from build123d import *
from OCP.BRepFilletAPI import BRepFilletAPI_MakeChamfer

# Parameters (mm, degrees)
BOSS_EXTRUDE1_DEPTH         = 2.29
SKETCH3_W                   = 0.64
SKETCH3_H                   = 0.64
CHAMFER3_SIZE               = 0.5
CHAMFER3_SIZE2              = 0.133974596
LPATTERN1_COUNT             = 6
LPATTERN1_PITCH             = 2.54
CHAMFER3_OF_LPATTERN1_SIZE  = 0.5
CHAMFER3_OF_LPATTERN1_SIZE2 = 0.133974596


with BuildPart() as part:
    # Sketch1 → Boss-Extrude1 (new body)
    with BuildSketch(Plane(origin=(0, 0, 0), x_dir=(1, 0, 0), z_dir=(0, 1, 0))):
        Polygon((-0.77, 1.25), (0.77, 1.25), (1.25, 0.75), (1.27, 0.75), (1.27, -0.75), (1.25, -0.75), (0.77, -1.25), (-0.77, -1.25), (-1.25, -0.75), (-1.27, -0.75), (-1.27, 0.75), (-1.25, 0.75), align=None)
    boss_extrude1 = extrude(amount=BOSS_EXTRUDE1_DEPTH)

    # Sweep1: sweep along a path in Sketch2
    with BuildLine(Plane(origin=(0, 0, 0), x_dir=(0, 0, -1), z_dir=(1, 0, 0))) as sweep1_path:
        Line((0, 17.12), (0, -0.408142235))
        ThreePointArc((0, -0.408142235), (-0.152240935, -1.1735091), (-0.585786438, -1.822355798))
        Line((-0.585786438, -1.822355798), (-5.26343064, -6.5))
    # Sketch3 → Sweep1 (sweep)
    with BuildSketch(Plane(origin=(0, 17.12, 0), x_dir=(1, 0, 0), z_dir=(0, 1, 0))):
        Rectangle(SKETCH3_W, SKETCH3_H)
    sweep1 = sweep(path=sweep1_path.line)

    # Chamfer3: one chamfer whose edges measure the first distance from different faces: ONE call of the kernel's chamfer builder (chamfer() names one face for all edges)
    chamfer3_edges_1 = [part.edges().sort_by_distance(p)[0] for p in [
        (0.32, 17.12, 0),
    ]]
    chamfer3_side_1 = [part.faces().sort_by_distance(p)[0] for p in [
        (0.32, 9.705, 0),
    ]]
    chamfer3_edges_2 = [part.edges().sort_by_distance(p)[0] for p in [
        (0, 17.12, -0.32),
    ]]
    chamfer3_side_2 = [part.faces().sort_by_distance(p)[0] for p in [
        (0, 9.705, -0.32),
    ]]
    chamfer3_edges_3 = [part.edges().sort_by_distance(p)[0] for p in [
        (-0.32, 17.12, 0),
    ]]
    chamfer3_side_3 = [part.faces().sort_by_distance(p)[0] for p in [
        (-0.32, 9.705, 0),
    ]]
    chamfer3_edges_4 = [part.edges().sort_by_distance(p)[0] for p in [
        (0, 17.12, 0.32),
    ]]
    chamfer3_side_4 = [part.faces().sort_by_distance(p)[0] for p in [
        (0, 9.705, 0.32),
    ]]
    chamfer3 = BRepFilletAPI_MakeChamfer(part.part.solid().wrapped)
    for e in chamfer3_edges_1:
        chamfer3.Add(CHAMFER3_SIZE, CHAMFER3_SIZE2, e.wrapped, chamfer3_side_1[0].wrapped)  # the first distance lies on this face
    for e in chamfer3_edges_2:
        chamfer3.Add(CHAMFER3_SIZE, CHAMFER3_SIZE2, e.wrapped, chamfer3_side_2[0].wrapped)  # the first distance lies on this face
    for e in chamfer3_edges_3:
        chamfer3.Add(CHAMFER3_SIZE, CHAMFER3_SIZE2, e.wrapped, chamfer3_side_3[0].wrapped)  # the first distance lies on this face
    for e in chamfer3_edges_4:
        chamfer3.Add(CHAMFER3_SIZE, CHAMFER3_SIZE2, e.wrapped, chamfer3_side_4[0].wrapped)  # the first distance lies on this face
    add(Compound.cast(chamfer3.Shape()), mode=Mode.REPLACE)

    # LPattern1: Boss-Extrude1, Sweep1 ×6
    with Locations(*[(i * LPATTERN1_PITCH, 0, 0) for i in range(1, LPATTERN1_COUNT)]):
        add(boss_extrude1)
        add(sweep1)

    # Chamfer3 of LPattern1: one chamfer whose edges measure the first distance from different faces: ONE call of the kernel's chamfer builder (chamfer() names one face for all edges)
    chamfer3_of_lpattern1_edges_1 = [part.edges().sort_by_distance(p)[0] for p in [
        (2.86, 17.12, 0),
    ]]
    chamfer3_of_lpattern1_side_1 = [part.faces().sort_by_distance(p)[0] for p in [
        (2.86, 9.705, 0),
    ]]
    chamfer3_of_lpattern1_edges_2 = [part.edges().sort_by_distance(p)[0] for p in [
        (2.54, 17.12, -0.32),
    ]]
    chamfer3_of_lpattern1_side_2 = [part.faces().sort_by_distance(p)[0] for p in [
        (2.54, 9.705, -0.32),
    ]]
    chamfer3_of_lpattern1_edges_3 = [part.edges().sort_by_distance(p)[0] for p in [
        (2.22, 17.12, 0),
    ]]
    chamfer3_of_lpattern1_side_3 = [part.faces().sort_by_distance(p)[0] for p in [
        (2.22, 9.705, 0),
    ]]
    chamfer3_of_lpattern1_edges_4 = [part.edges().sort_by_distance(p)[0] for p in [
        (2.54, 17.12, 0.32),
    ]]
    chamfer3_of_lpattern1_side_4 = [part.faces().sort_by_distance(p)[0] for p in [
        (2.54, 9.705, 0.32),
    ]]
    chamfer3_of_lpattern1_edges_5 = [part.edges().sort_by_distance(p)[0] for p in [
        (5.4, 17.12, 0),
    ]]
    chamfer3_of_lpattern1_side_5 = [part.faces().sort_by_distance(p)[0] for p in [
        (5.4, 9.705, 0),
    ]]
    chamfer3_of_lpattern1_edges_6 = [part.edges().sort_by_distance(p)[0] for p in [
        (5.08, 17.12, -0.32),
    ]]
    chamfer3_of_lpattern1_side_6 = [part.faces().sort_by_distance(p)[0] for p in [
        (5.08, 9.705, -0.32),
    ]]
    chamfer3_of_lpattern1_edges_7 = [part.edges().sort_by_distance(p)[0] for p in [
        (4.76, 17.12, 0),
    ]]
    chamfer3_of_lpattern1_side_7 = [part.faces().sort_by_distance(p)[0] for p in [
        (4.76, 9.705, 0),
    ]]
    chamfer3_of_lpattern1_edges_8 = [part.edges().sort_by_distance(p)[0] for p in [
        (5.08, 17.12, 0.32),
    ]]
    chamfer3_of_lpattern1_side_8 = [part.faces().sort_by_distance(p)[0] for p in [
        (5.08, 9.705, 0.32),
    ]]
    chamfer3_of_lpattern1_edges_9 = [part.edges().sort_by_distance(p)[0] for p in [
        (7.94, 17.12, 0),
    ]]
    chamfer3_of_lpattern1_side_9 = [part.faces().sort_by_distance(p)[0] for p in [
        (7.94, 9.705, 0),
    ]]
    chamfer3_of_lpattern1_edges_10 = [part.edges().sort_by_distance(p)[0] for p in [
        (7.62, 17.12, -0.32),
    ]]
    chamfer3_of_lpattern1_side_10 = [part.faces().sort_by_distance(p)[0] for p in [
        (7.62, 9.705, -0.32),
    ]]
    chamfer3_of_lpattern1_edges_11 = [part.edges().sort_by_distance(p)[0] for p in [
        (7.3, 17.12, 0),
    ]]
    chamfer3_of_lpattern1_side_11 = [part.faces().sort_by_distance(p)[0] for p in [
        (7.3, 9.705, 0),
    ]]
    chamfer3_of_lpattern1_edges_12 = [part.edges().sort_by_distance(p)[0] for p in [
        (7.62, 17.12, 0.32),
    ]]
    chamfer3_of_lpattern1_side_12 = [part.faces().sort_by_distance(p)[0] for p in [
        (7.62, 9.705, 0.32),
    ]]
    chamfer3_of_lpattern1_edges_13 = [part.edges().sort_by_distance(p)[0] for p in [
        (10.48, 17.12, 0),
    ]]
    chamfer3_of_lpattern1_side_13 = [part.faces().sort_by_distance(p)[0] for p in [
        (10.48, 9.705, 0),
    ]]
    chamfer3_of_lpattern1_edges_14 = [part.edges().sort_by_distance(p)[0] for p in [
        (10.16, 17.12, -0.32),
    ]]
    chamfer3_of_lpattern1_side_14 = [part.faces().sort_by_distance(p)[0] for p in [
        (10.16, 9.705, -0.32),
    ]]
    chamfer3_of_lpattern1_edges_15 = [part.edges().sort_by_distance(p)[0] for p in [
        (9.84, 17.12, 0),
    ]]
    chamfer3_of_lpattern1_side_15 = [part.faces().sort_by_distance(p)[0] for p in [
        (9.84, 9.705, 0),
    ]]
    chamfer3_of_lpattern1_edges_16 = [part.edges().sort_by_distance(p)[0] for p in [
        (10.16, 17.12, 0.32),
    ]]
    chamfer3_of_lpattern1_side_16 = [part.faces().sort_by_distance(p)[0] for p in [
        (10.16, 9.705, 0.32),
    ]]
    chamfer3_of_lpattern1_edges_17 = [part.edges().sort_by_distance(p)[0] for p in [
        (13.02, 17.12, 0),
    ]]
    chamfer3_of_lpattern1_side_17 = [part.faces().sort_by_distance(p)[0] for p in [
        (13.02, 9.705, 0),
    ]]
    chamfer3_of_lpattern1_edges_18 = [part.edges().sort_by_distance(p)[0] for p in [
        (12.7, 17.12, -0.32),
    ]]
    chamfer3_of_lpattern1_side_18 = [part.faces().sort_by_distance(p)[0] for p in [
        (12.7, 9.705, -0.32),
    ]]
    chamfer3_of_lpattern1_edges_19 = [part.edges().sort_by_distance(p)[0] for p in [
        (12.38, 17.12, 0),
    ]]
    chamfer3_of_lpattern1_side_19 = [part.faces().sort_by_distance(p)[0] for p in [
        (12.38, 9.705, 0),
    ]]
    chamfer3_of_lpattern1_edges_20 = [part.edges().sort_by_distance(p)[0] for p in [
        (12.7, 17.12, 0.32),
    ]]
    chamfer3_of_lpattern1_side_20 = [part.faces().sort_by_distance(p)[0] for p in [
        (12.7, 9.705, 0.32),
    ]]
    chamfer3_of_lpattern1 = BRepFilletAPI_MakeChamfer(part.part.solid().wrapped)
    for e in chamfer3_of_lpattern1_edges_1:
        chamfer3_of_lpattern1.Add(CHAMFER3_OF_LPATTERN1_SIZE, CHAMFER3_OF_LPATTERN1_SIZE2, e.wrapped, chamfer3_of_lpattern1_side_1[0].wrapped)  # the first distance lies on this face
    for e in chamfer3_of_lpattern1_edges_2:
        chamfer3_of_lpattern1.Add(CHAMFER3_OF_LPATTERN1_SIZE, CHAMFER3_OF_LPATTERN1_SIZE2, e.wrapped, chamfer3_of_lpattern1_side_2[0].wrapped)  # the first distance lies on this face
    for e in chamfer3_of_lpattern1_edges_3:
        chamfer3_of_lpattern1.Add(CHAMFER3_OF_LPATTERN1_SIZE, CHAMFER3_OF_LPATTERN1_SIZE2, e.wrapped, chamfer3_of_lpattern1_side_3[0].wrapped)  # the first distance lies on this face
    for e in chamfer3_of_lpattern1_edges_4:
        chamfer3_of_lpattern1.Add(CHAMFER3_OF_LPATTERN1_SIZE, CHAMFER3_OF_LPATTERN1_SIZE2, e.wrapped, chamfer3_of_lpattern1_side_4[0].wrapped)  # the first distance lies on this face
    for e in chamfer3_of_lpattern1_edges_5:
        chamfer3_of_lpattern1.Add(CHAMFER3_OF_LPATTERN1_SIZE, CHAMFER3_OF_LPATTERN1_SIZE2, e.wrapped, chamfer3_of_lpattern1_side_5[0].wrapped)  # the first distance lies on this face
    for e in chamfer3_of_lpattern1_edges_6:
        chamfer3_of_lpattern1.Add(CHAMFER3_OF_LPATTERN1_SIZE, CHAMFER3_OF_LPATTERN1_SIZE2, e.wrapped, chamfer3_of_lpattern1_side_6[0].wrapped)  # the first distance lies on this face
    for e in chamfer3_of_lpattern1_edges_7:
        chamfer3_of_lpattern1.Add(CHAMFER3_OF_LPATTERN1_SIZE, CHAMFER3_OF_LPATTERN1_SIZE2, e.wrapped, chamfer3_of_lpattern1_side_7[0].wrapped)  # the first distance lies on this face
    for e in chamfer3_of_lpattern1_edges_8:
        chamfer3_of_lpattern1.Add(CHAMFER3_OF_LPATTERN1_SIZE, CHAMFER3_OF_LPATTERN1_SIZE2, e.wrapped, chamfer3_of_lpattern1_side_8[0].wrapped)  # the first distance lies on this face
    for e in chamfer3_of_lpattern1_edges_9:
        chamfer3_of_lpattern1.Add(CHAMFER3_OF_LPATTERN1_SIZE, CHAMFER3_OF_LPATTERN1_SIZE2, e.wrapped, chamfer3_of_lpattern1_side_9[0].wrapped)  # the first distance lies on this face
    for e in chamfer3_of_lpattern1_edges_10:
        chamfer3_of_lpattern1.Add(CHAMFER3_OF_LPATTERN1_SIZE, CHAMFER3_OF_LPATTERN1_SIZE2, e.wrapped, chamfer3_of_lpattern1_side_10[0].wrapped)  # the first distance lies on this face
    for e in chamfer3_of_lpattern1_edges_11:
        chamfer3_of_lpattern1.Add(CHAMFER3_OF_LPATTERN1_SIZE, CHAMFER3_OF_LPATTERN1_SIZE2, e.wrapped, chamfer3_of_lpattern1_side_11[0].wrapped)  # the first distance lies on this face
    for e in chamfer3_of_lpattern1_edges_12:
        chamfer3_of_lpattern1.Add(CHAMFER3_OF_LPATTERN1_SIZE, CHAMFER3_OF_LPATTERN1_SIZE2, e.wrapped, chamfer3_of_lpattern1_side_12[0].wrapped)  # the first distance lies on this face
    for e in chamfer3_of_lpattern1_edges_13:
        chamfer3_of_lpattern1.Add(CHAMFER3_OF_LPATTERN1_SIZE, CHAMFER3_OF_LPATTERN1_SIZE2, e.wrapped, chamfer3_of_lpattern1_side_13[0].wrapped)  # the first distance lies on this face
    for e in chamfer3_of_lpattern1_edges_14:
        chamfer3_of_lpattern1.Add(CHAMFER3_OF_LPATTERN1_SIZE, CHAMFER3_OF_LPATTERN1_SIZE2, e.wrapped, chamfer3_of_lpattern1_side_14[0].wrapped)  # the first distance lies on this face
    for e in chamfer3_of_lpattern1_edges_15:
        chamfer3_of_lpattern1.Add(CHAMFER3_OF_LPATTERN1_SIZE, CHAMFER3_OF_LPATTERN1_SIZE2, e.wrapped, chamfer3_of_lpattern1_side_15[0].wrapped)  # the first distance lies on this face
    for e in chamfer3_of_lpattern1_edges_16:
        chamfer3_of_lpattern1.Add(CHAMFER3_OF_LPATTERN1_SIZE, CHAMFER3_OF_LPATTERN1_SIZE2, e.wrapped, chamfer3_of_lpattern1_side_16[0].wrapped)  # the first distance lies on this face
    for e in chamfer3_of_lpattern1_edges_17:
        chamfer3_of_lpattern1.Add(CHAMFER3_OF_LPATTERN1_SIZE, CHAMFER3_OF_LPATTERN1_SIZE2, e.wrapped, chamfer3_of_lpattern1_side_17[0].wrapped)  # the first distance lies on this face
    for e in chamfer3_of_lpattern1_edges_18:
        chamfer3_of_lpattern1.Add(CHAMFER3_OF_LPATTERN1_SIZE, CHAMFER3_OF_LPATTERN1_SIZE2, e.wrapped, chamfer3_of_lpattern1_side_18[0].wrapped)  # the first distance lies on this face
    for e in chamfer3_of_lpattern1_edges_19:
        chamfer3_of_lpattern1.Add(CHAMFER3_OF_LPATTERN1_SIZE, CHAMFER3_OF_LPATTERN1_SIZE2, e.wrapped, chamfer3_of_lpattern1_side_19[0].wrapped)  # the first distance lies on this face
    for e in chamfer3_of_lpattern1_edges_20:
        chamfer3_of_lpattern1.Add(CHAMFER3_OF_LPATTERN1_SIZE, CHAMFER3_OF_LPATTERN1_SIZE2, e.wrapped, chamfer3_of_lpattern1_side_20[0].wrapped)  # the first distance lies on this face
    add(Compound.cast(chamfer3_of_lpattern1.Shape()), mode=Mode.REPLACE)


solid = part.part
Input: part model. Units: mm. Frame: model coordinates. A direction names the side the tool comes from. Give positions to 0.01 mm unless a question says otherwise; leave off trailing zeros. Order: outer loops, then holes, each group sorted by start corner. A loop starts at its lowest first (then second) coordinate and runs counter-clockwise, first axis right, second up.
Q1. Ray query, probe 1 along X at (y, z) = (7.25, -0.25); probe 2 along X at (y, z) = (1.5, -1); probe 3 along Z at (x, y) = (8.25, 0.5). Return the intervals inside material, ascending.
Checked values:
probe 1: x = -0.32 to 0.32, 2.22 to 2.86, 4.76 to 5.4, 7.3 to 7.94, 9.84 to 10.48, 12.38 to 13.02
probe 2: x = -1.01 to 1.01, 1.53 to 3.55, 4.07 to 6.09, 6.61 to 8.63, 9.15 to 11.17, 11.69 to 13.71
probe 3: z = -1.25 to 1.25
Q2. Section B-B on z = 1.75. Output: boundary loops of the cut face in (x, y), and give its area (3 significant figures).
Checked values:
outline: (-0.32, -3.44) - (0.32, -3.44) - (0.32, -2.53) - (-0.32, -2.53) - close; (2.22, -3.44) - (2.86, -3.44) - (2.86, -2.53) - (2.22, -2.53) - close; (4.76, -3.44) - (5.4, -3.44) - (5.4, -2.53) - (4.76, -2.53) - close; (7.3, -3.44) - (7.94, -3.44) - (7.94, -2.53) - (7.3, -2.53) - close; (9.84, -3.44) - (10.48, -3.44) - (10.48, -2.53) - (9.84, -2.53) - close; (12.38, -3.44) - (13.02, -3.44) - (13.02, -2.53) - (12.38, -2.53) - close
area: 3.48 mm2
Q3. Set-up query: faces 1 (the flat face through (8, 1, -1.25)), 2 (the flat face through (13.02, -3, 2)), 3 (the flat face through (0, 1, 1.25)), 4 (the flat face through (2.22, -3, 2)). Return all of +Z, -Z, +X, -X, +Y, -Y with unobstructed straight access to the full face (end or side cutting, diameter ignored); none if empty.
Checked values:
face 1: -Z, +X, -X, +Y, -Y
face 2: +Z, -Z, +X, -Y
face 3: +Z, +X, -X, +Y
face 4: +Z, -Z, -Y
Q4. Contact query for flat-ended pins moving along their axis: pin 1 Ø4 at (x, y) = (4, 6.5) entering from -Z; pin 2 Ø1.7 at (y, z) = (-3.5, 3) entering from +X. Output: stop coordinate, or through.
Checked values:
pin 1: stops at z = -0.32
pin 2: stops at x = 13.02
Q5. Section A-A on y = 7.25. Output: boundary loops of the cut face in (x, z).
Checked values:
outline: (-0.32, -0.32) - (0.32, -0.32) - (0.32, 0.32) - (-0.32, 0.32) - close; (2.22, -0.32) - (2.86, -0.32) - (2.86, 0.32) - (2.22, 0.32) - close; (4.76, -0.32) - (5.4, -0.32) - (5.4, 0.32) - (4.76, 0.32) - close; (7.3, -0.32) - (7.94, -0.32) - (7.94, 0.32) - (7.3, 0.32) - close; (9.84, -0.32) - (10.48, -0.32) - (10.48, 0.32) - (9.84, 0.32) - close; (12.38, -0.32) - (13.02, -0.32) - (13.02, 0.32) - (12.38, 0.32) - close
Q6. Draft query along Y for faces 5 (the flat face through (6, 0, 0)), 6 (the flat face through (5.08, -4.42, 2.73)), 7 (the flat face through (13, 1, -1.25)). Return one class per face: +Y half, -Y half, draft (parallel to the pull), parting line (faces both ways), or undercut.
Checked values:
face 5: undercut
face 6: -Y half
face 7: draft
